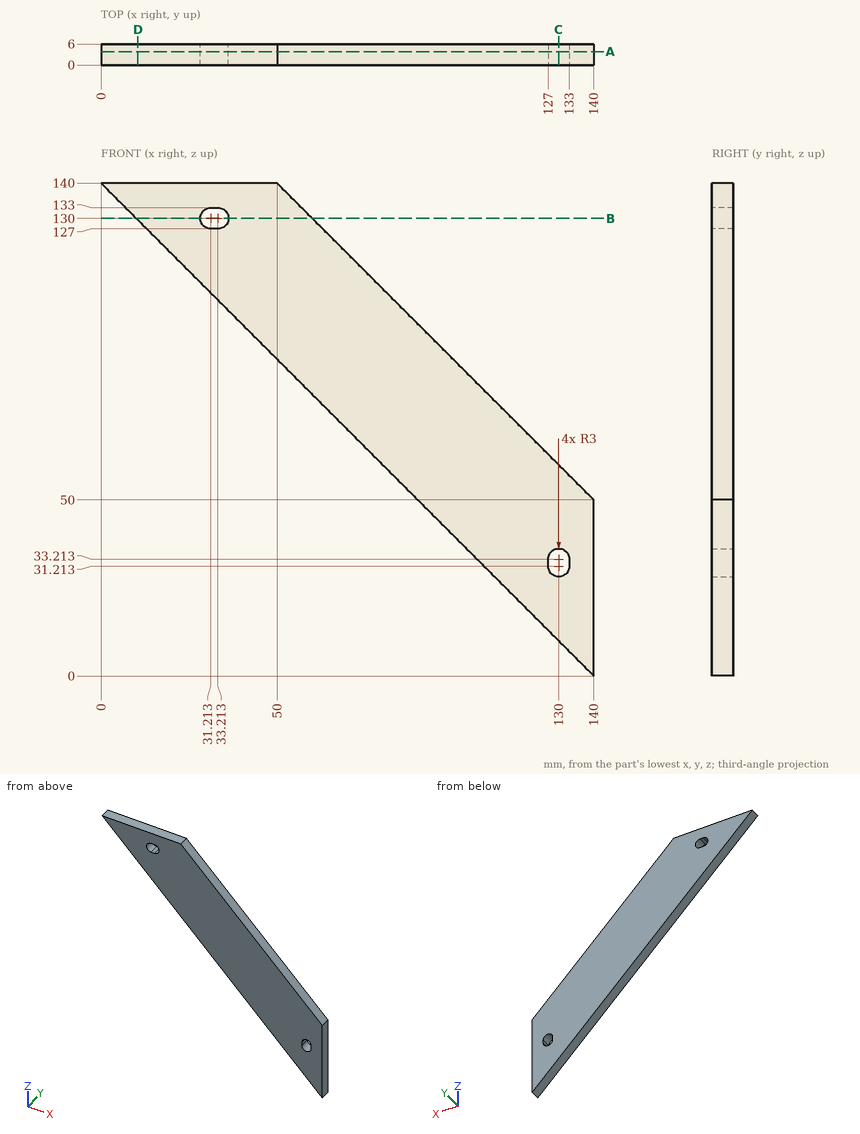
Could you check a few things on this drawing? It's one solid part, dimensions in mm from its lowest x, y, z. Give positions to 0.01 mm unless a question says otherwise; leave off trailing zeros. Write each loop counter-clockwise with the first axis right and the second up, starting at its lowest first coordinate (ties: lowest second). Pieces come first, ordered by that corner, then holes. Notation, with made-up numbers: (9.5, 4) -> (48.5, 4) arc R30 cw to (48.5, 32) -> close; hole circle Ø3 at (-4.5, 52). An arc over 180 degrees is marked (long way). Answer as CSV lines item,"result". Start each with the question number.
(1) If we section it at A-A, the plane y = 3.8: Write out the boundary of the cut face in (x, z), and give its area (3 significant figures).
(2) Please list where these lines run through material, in increasing order: line 1 (X direction, y = 3.6, z = 132.5) (1 decimal); line 2 (Z direction, x = 97.5, y = 4.1); line 3 (X direction, y = 0.95, z = 12.5).
(3) If we section it at D-D, the plane x = 10.5: Write out the boundary of the cut face in (y, z), and give its area (3 significant figures).
(4) If we section it at B-B, the plane z = 130: Write out the boundary of the cut face in (x, y).
(5) If we section it at C-C, the plane x = 130: Write out the boundary of the cut face in (y, z), and give its area (3 significant figures).
(6) I'm going to push flat-ended pins straight in: pin 1 Ø3 at (x, y) = (116, 1.5) entering from -Z; pin 2 Ø2 at (x, y) = (32, 2.5) entering from -Z; pin 3 Ø2 at (y, z) = (5.5, 69) entering from -X. Where does each tip first touch, or does it pass through?
Answer list:
1,outline,"(0, 140) -> (140, 0) -> (140, 50) -> (50, 140) -> close; hole (31.21, 127) -> (33.21, 127) arc R3 ccw to (33.21, 133) -> (31.21, 133) arc R3 ccw to start; hole (127, 31.21) arc R3 ccw to (133, 31.21) -> (133, 33.21) arc R3 ccw to (127, 33.21) -> close"
1,area,"5,670 mm^2"
2,line 1,"7.5 to 29.6, 34.9 to 57.5"
2,line 2,"42.5 to 92.5"
2,line 3,"127.5 to 140"
3,outline,"(0, 129.5) -> (6, 129.5) -> (6, 140) -> (0, 140) -> close"
3,area,"63.0 mm^2"
4,outline,"(10, 0) -> (28.21, 0) -> (28.21, 6) -> (10, 6) -> close; (36.21, 0) -> (60, 0) -> (60, 6) -> (36.21, 6) -> close"
5,outline,"(0, 10) -> (6, 10) -> (6, 28.21) -> (0, 28.21) -> close; (0, 36.21) -> (6, 36.21) -> (6, 60) -> (0, 60) -> close"
5,area,"252 mm^2"
6,pin 1,"z = 22.5"
6,pin 2,"z = 107"
6,pin 3,"x = 70"
